Verification items for the finished model (mm, model axes). A direction names the side the tool comes from. Round coordinates to 2 decimals unless told otherwise and drop trailing zeros. Write each loop counter-clockwise with the first axis right and the second up, starting at its lowest first coordinate (ties: lowest second). Pieces come first, ordered by that corner, then holes. Notation, with made-up numbers: (73.5, 83) - (81.5, 83) arc R13 ccw to (81.5, 99) - close; hole circle Ø6 at (59.5, 57). An arc over 180 degrees is marked (long way). Write each question's results on one line, items separated by ' | '.
```python
from build123d import *

# Parameters (mm, degrees)
CROQUIS1_R              = 2.6
SALIENTE_EXTRUIR1_DEPTH = 10
REDONDEO1_R             = 0.2
REDONDEO2_R             = 0.1


with BuildPart() as part:
    # Croquis1 → Saliente-Extruir1 (new body)
    with BuildSketch(Plane.YZ):
        Polygon((5, -10), (5, 10), (0, 5.00000025), (-5, 10), (-5, -10), (0, -4.99999975), align=None)
        with Locations(Location((0, 0, 0), (0, 0, 270))):
            Circle(CROQUIS1_R, mode=Mode.SUBTRACT)
    extrude(amount=SALIENTE_EXTRUIR1_DEPTH)

    # Redondeo1
    redondeo1_edges = [part.edges().sort_by_distance(p)[0] for p in [
        (5, 0, -4.99999975),
        (5, -5, -10),
        (5, -5, 10),
        (5, 0, 5.00000025),
        (5, 5, 10),
        (5, 5, -10),
    ]]
    fillet(redondeo1_edges, radius=REDONDEO1_R)

    # Redondeo2
    redondeo2_edges = [part.edges().sort_by_distance(p)[0] for p in [
        (0, 0, 2.6),
        (10, 0, 2.6),
    ]]
    fillet(redondeo2_edges, radius=REDONDEO2_R)


solid = part.part
```
(1) Thickness scan on L1, parallel to Y at x = 8, z = 0; L2, parallel to Y at x = 7, z = -8.5; L3, parallel to Z at x = 3.5, y = 0.75. Record the ranges inside material, lowest first.
Answer:
L1: -5 to -2.6, 2.6 to 5 | L2: -5 to -3.5, 3.5 to 5 | L3: -5.75 to -2.49, 2.49 to 5.75
(2) Section check A-A (z = 0). Record the cut outline in (x, y).
Answer:
outline: (0, -5) - (10, -5) - (10, -2.7) arc R0.1 ccw to (9.9, -2.6) - (0.1, -2.6) arc R0.1 ccw to (0, -2.7) - close; (0, 2.7) arc R0.1 ccw to (0.1, 2.6) - (9.9, 2.6) arc R0.1 ccw to (10, 2.7) - (10, 5) - (0, 5) - close
(3) Section check B-B (x = 6.25). Record the cut outline in (y, z), plus the area to 3 significant figures.
Answer:
outline: (-5, -9.52) arc R0.2 ccw to (-4.66, -9.66) - (-0.14, -5.14) arc R0.2 cw to (0.14, -5.14) - (4.66, -9.66) arc R0.2 ccw to (5, -9.52) - (5, 9.52) arc R0.2 ccw to (4.66, 9.66) - (0.14, 5.14) arc R0.2 cw to (-0.14, 5.14) - (-4.66, 9.66) arc R0.2 ccw to (-5, 9.52) - close; hole circle Ø5.2 at (0, 0) | area: 129 mm2
(4) Set-up check for faces 1 (the flat face through (5, 2, 7)), 2 (the flat face through (5, -2, -7)), 3 (the flat face through (5, 5, 0)): record each of +Z, -Z, +X, -X, +Y, -Y from which the full face is reachable in a straight line by a thin tool's end or side.
Answer:
face 1: +Z, +X, -X | face 2: -Z, +X, -X | face 3: +Z, -Z, +X, -X, +Y
(5) Section check C-C (z = 6.5). Record the cut outline in (x, y), plus the area to 3 significant figures.
Answer:
outline: (0, -5) - (10, -5) - (10, -1.5) - (0, -1.5) - close; (0, 1.5) - (10, 1.5) - (10, 5) - (0, 5) - close | area: 70.0 mm2
(6) Section check D-D (y = 3.5). Record the cut outline in (x, z), plus the area to 3 significant figures.
Answer:
outline: (0, -8.5) - (10, -8.5) - (10, 8.5) - (0, 8.5) - close | area: 170 mm2
(7) Mould release check, pull along Y, two halves, no side actions. Record for faces 4 (the flat face through (5, -2, 7)), 5 (the flat face through (5, -5, 0)), 6 (the flat face through (10, 2.2, 2.3)): released by +Y, released by -Y, zero draft, split by the parting line, or undercut.
Answer:
face 4: undercut | face 5: released by -Y | face 6: zero draft
(8) Go/stop test with flat-tipped pins: pin 1 Ø4 at (x, y) = (7.5, -1.5) entering from +Z; pin 2 Ø1.5 at (x, y) = (5.5, 3.5) entering from +Z; pin 3 Ø4 at (x, y) = (2, 0) entering from -Z; pin 4 Ø4.5 at (y, z) = (0, 0) entering from -X. Record where each tip stops, or that it passes through.
Answer:
pin 1: z = 8.5 | pin 2: z = 9.25 | pin 3: z = -7 | pin 4: through
